```python
from build123d import *

# Parameters (mm, degrees)
F0_R      = 26
F0_W      = 24
F0_H      = 18
F1_DEPTH  = 11
F3_DEPTH  = 2
F4_W      = 26
F4_H      = 20
F5_DEPTH  = 7
F6_W      = 28
F6_H      = 22
F7_DEPTH  = 6
F8_W      = 30
F8_H      = 24
F9_DEPTH  = 5
F10_W     = 32
F10_H     = 26
F11_DEPTH = 4
F12_DEPTH = 4
F13_W     = 34
F13_H     = 28
F14_DEPTH = 3
F15_W     = 36
F15_H     = 30
F15_W_2   = 34
F15_H_2   = 28
F16_DEPTH = 2
F17_W     = 38
F17_H     = 32
F17_W_2   = 36
F17_H_2   = 30
F18_DEPTH = 1
F19_R     = 1
F20_R     = 1.5
F21_DEPTH = 25
F22_R     = 2.5
F23_DEPTH = 5


with BuildPart() as f1:
    # F0 (on Front) → F1 (new body)
    with BuildSketch(Plane.XZ):
        Circle(F0_R)
        Rectangle(F0_W, F0_H, mode=Mode.SUBTRACT)
    extrude(amount=F1_DEPTH)

    # F2 (on face) → F3 (cut)
    with BuildSketch(Plane(origin=(0, 0, 0), x_dir=(-1, 0, 0), z_dir=(0, 1, 0))):
        with BuildLine():
            ThreePointArc((14, 9), (13.4142135624, 10.4142135624), (12, 11))
            Line((12, 11), (-12, 11))
            ThreePointArc((-12, 11), (-13.4142135624, 10.4142135624), (-14, 9))
            Line((-14, 9), (-14, -9))
            ThreePointArc((-14, -9), (-13.4142135624, -10.4142135624), (-12, -11))
            Line((-12, -11), (12, -11))
            ThreePointArc((12, -11), (13.4142135624, -10.4142135624), (14, -9))
            Line((14, -9), (14, 9))
        make_face()
    extrude(amount=-F3_DEPTH, mode=Mode.SUBTRACT)

    # F4 (on face) → F5 (cut)
    with BuildSketch(Plane.XZ.offset(11)):
        Rectangle(F4_W, F4_H)
    extrude(amount=-F5_DEPTH, mode=Mode.SUBTRACT)

    # F6 (on face) → F7 (cut)
    with BuildSketch(Plane.XZ.offset(11)):
        Rectangle(F6_W, F6_H)
    extrude(amount=-F7_DEPTH, mode=Mode.SUBTRACT)

    # F8 (on face) → F9 (cut)
    with BuildSketch(Plane.XZ.offset(11)):
        Rectangle(F8_W, F8_H)
    extrude(amount=-F9_DEPTH, mode=Mode.SUBTRACT)

    # F10 (on face) → F11 (cut)
    with BuildSketch(Plane.XZ.offset(11)):
        Rectangle(F10_W, F10_H)
    extrude(amount=-F11_DEPTH, mode=Mode.SUBTRACT)

    # F10 (on face) → F12 (cut)
    with BuildSketch(Plane.XZ.offset(11)):
        Rectangle(F10_W, F10_H)
    extrude(amount=-F12_DEPTH, mode=Mode.SUBTRACT)

    # F13 (on face) → F14 (cut)
    with BuildSketch(Plane.XZ.offset(11)):
        Rectangle(F13_W, F13_H)
    extrude(amount=-F14_DEPTH, mode=Mode.SUBTRACT)

    # F15 (on face) → F16 (cut)
    with BuildSketch(Plane.XZ.offset(11)):
        Rectangle(F15_W, F15_H)
        Rectangle(F15_W_2, F15_H_2, mode=Mode.SUBTRACT)
    extrude(amount=-F16_DEPTH, mode=Mode.SUBTRACT)

    # F17 (on face) → F18 (cut)
    with BuildSketch(Plane.XZ.offset(11)):
        Rectangle(F17_W, F17_H)
        Rectangle(F17_W_2, F17_H_2, mode=Mode.SUBTRACT)
    extrude(amount=-F18_DEPTH, mode=Mode.SUBTRACT)

    # F19
    f19_edges = [f1.edges().sort_by_distance(p)[0] for p in [
        (15, -6.5, -12),
        (13, -4.5, -10),
        (14, -5.5, -11),
        (12, -3, -9),
        (-15, -6.5, -12),
        (-14, -5.5, -11),
        (-13, -4.5, -10),
        (-12, -3, -9),
        (-12, -3, 9),
        (-13, -4.5, 10),
        (-14, -5.5, 11),
        (-15, -6.5, 12),
        (15, -6.5, 12),
        (14, -5.5, 11),
        (12, -3, 9),
        (13, -4.5, 10),
        (16, -7.5, -13),
        (17, -8.5, -14),
        (18, -9.5, -15),
        (19, -10.5, -16),
        (-16, -7.5, -13),
        (-17, -8.5, -14),
        (-18, -9.5, -15),
        (-19, -10.5, -16),
        (-16, -7.5, 13),
        (-17, -8.5, 14),
        (-18, -9.5, 15),
        (-19, -10.5, 16),
        (19, -10.5, 16),
        (18, -9.5, 15),
        (16, -7.5, 13),
        (17, -8.5, 14),
    ]]
    fillet(f19_edges, radius=F19_R)

    # F20 (on face) → F21 (cut)
    with BuildSketch(Plane.XZ.offset(11)):
        with Locations((-16, 0)):
            Circle(F20_R)
        with Locations((16, 0)):
            Circle(F20_R)
    extrude(amount=-F21_DEPTH, mode=Mode.SUBTRACT)

    # F22 (on face) → F23 (cut)
    with BuildSketch(Plane.XZ.offset(11)):
        with Locations((-16, 0)):
            Circle(F22_R)
        with Locations((16, 0)):
            Circle(F22_R)
    extrude(amount=-F23_DEPTH, mode=Mode.SUBTRACT)


solid = f1.part
```
The listing builds one solid part. Answer for the finished solid, in the listing's coordinates (mm). A direction names the side the tool comes from. Round coordinates to 2 decimals unless told otherwise and drop trailing zeros. Loops run counter-clockwise (first coordinate to the right, second up) from the corner with the lowest first, then second, coordinate; pieces in that order, holes last.
1) Given P1, Ø0.5, axis at y = -9.5, z = 7, coming from the +X side; P2, Ø5, axis at x = 17, y = -5.5, coming from the +Z side; P3, Ø0.5, axis at y = -8.5, z = -8.5, coming from the -X side; P4, Ø2.5, axis at x = 16, z = 0, coming from the -Y side, each flat-ended and moving along its own axis, determine where each tip first touches the part or whether it passes through.
Outcome:
P1: stops at x = 25.11
P2: stops at z = 21.58
P3: stops at x = -24.66
P4: passes through
2) For a pull along Z with two mould halves and no side action, classify faces 4 (the face through (-0.4, 0, -11.2)), 5 (the face through (0, -2, -10)), 6 (the face through (-20.633, -5.423, -15.821)), 7 (the face through (-0.1, -10, -15.3)) as released by +Z, released by -Z, zero draft, split by the parting line, or undercut.
Outcome:
face 4: zero draft
face 5: undercut
face 6: split by the parting line
face 7: undercut
3) A cutting plane is placed at A-A on z = 0. Give the number of separate pieces and of enclosed holes in the cut face, plus the area to 3 significant figures.
Outcome:
separate pieces: 4
enclosed holes: 0
area: 192 mm2
4) Consider line 1 (X direction, y = -2.5, z = 0.5); line 2 (Z direction, x = 0.5, y = -0.25); line 3 (Y direction, x = 16.5, z = -3). Determine where each line is inside the solid, lowest interval first.
Outcome:
line 1: x = -26 to -17.41, -14.59 to -12, 12 to 14.59, 17.41 to 26
line 2: z = -26 to -11, 11 to 26
line 3: y = -8 to 0
5) For faces 1 (the face through (14, -1, 0)), 2 (the face through (-18.5, -7.6, 0.1)), 3 (the face through (0, -3, 9)), determine the directions among +Z, -Z, +X, -X, +Y, -Y from which every point of the face is accessible in a straight line to the end or side of a thin tool.
Outcome:
face 1: +Y
face 2: -Y
face 3: +Y, -Y
6) A cutting plane is placed at B-B on z = -17. Determine the outline of the cut face in (x, y).
Outcome:
outline: (-19.67, -11) - (19.67, -11) - (19.67, 0) - (-19.67, 0) - close
